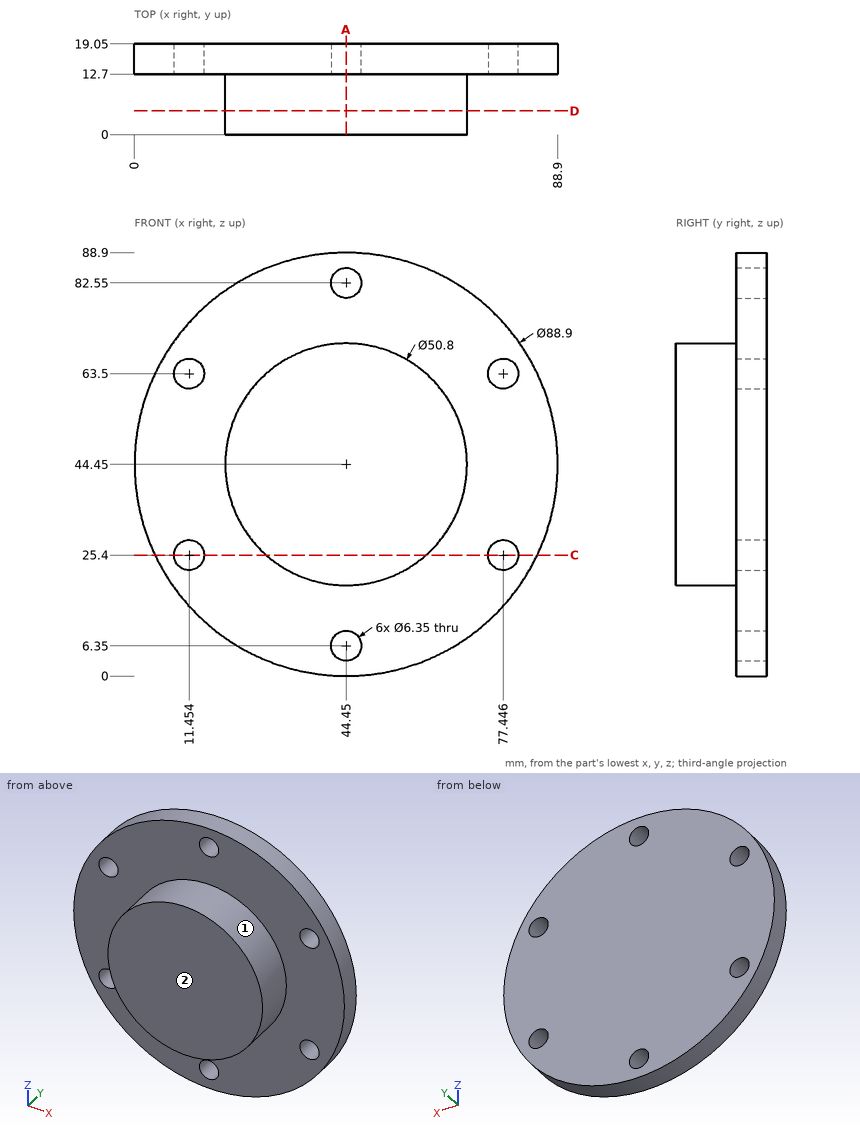
Design review of the part shown in the three views and the two pictorial views. Dimensions are in mm from the part's minimum x, y and z. A direction names the side the tool comes from. Coordinates: 2 decimals unless noted, no trailing zeros. Write each loop counter-clockwise with the first axis right and the second up, starting at its lowest first coordinate (ties: lowest second). Pieces come first, ordered by that corner, then holes.
(1) Add section C-C on z = 25.4. Give the boundary of the cut face in (x, y), then the cut area to 3 significant figures.
(2) Wall thickness on probe 1 along Z at (x, y) = (44.45, 14.75) (1 decimal); probe 2 along Y at (x, z) = (68, 21); probe 3 along X at (y, z) = (13.75, 81) (1 decimal): over which ranges is each line inside the solid? List them lowest first.
(3) Add section A-A on x = 44.45. Count the separate pieces of the cut face and the enclosed holes in it, then the cut area to 3 significant figures.
(4) Tool access review of the marked faces 1 and 2: name each direction out of +Z, -Z, +X, -X, +Y, -Y from which nothing blocks a thin tool from reaching the whole face with its end or side.
(5) Add section D-D on y = 5. Give the boundary of the cut face in (x, z).
(6) For pin 1 Ø5 at (x, y) = (35, 10.5) entering from +Z (1 decimal); pin 2 Ø8.5 at (x, z) = (77.45, 63.5) entering from -Y; pin 3 Ø8.5 at (x, z) = (44.45, 6.35) entering from +Y; pin 4 Ø2 at (x, y) = (49, 9) entering from -Z, all flat-tipped, find the tip position at first contact; note any pin that passes through.
Answer sheet:
1. outline: (4.29, 12.7) - (8.28, 12.7) - (8.28, 19.05) - (4.29, 19.05) - close; (14.63, 12.7) - (27.65, 12.7) - (27.65, 0) - (61.25, 0) - (61.25, 12.7) - (74.27, 12.7) - (74.27, 19.05) - (14.63, 19.05) - close; (80.62, 12.7) - (84.61, 12.7) - (84.61, 19.05) - (80.62, 19.05) - close
1. area: 856 mm2
2. probe 1: z = 0 to 3.2, 9.5 to 79.4, 85.7 to 88.9
2. probe 2: y = 12.7 to 19.05
2. probe 3: x = 19.2 to 41.7, 47.2 to 69.7
3. separate pieces: 3
3. enclosed holes: 0
3. area: 1,130 mm2
4. face 1: -Y
4. face 2: +Z, -Z, +X, -X, -Y
5. outline: circle Ø50.8 at (44.45, 44.45)
6. pin 1: stops at z = 88.1
6. pin 2: stops at y = 12.7
6. pin 3: stops at y = 19.05
6. pin 4: stops at z = 19.3
